Here's how the part is built. I have some questions about the finished solid (model axes, mm). Face numbers are marked on the shaded views. A direction names the side the tool comes from. Round coordinates to 2 decimals unless told otherwise and drop trailing zeros. Loops run counter-clockwise (first coordinate to the right, second up) from the corner with the lowest first, then second, coordinate; pieces in that order, holes last. Notation, with made-up numbers: (0.5, 5) -> (50.5, 5) arc R30 ccw to (50.5, 36) -> close; hole circle Ø8 at (45.5, 50.25). An arc over 180 degrees is marked (long way). One line per item, written item: value. Start each with the question number.
```python
from build123d import *

# Parameters (mm, degrees)
SKETCH2_R               = 4.3
SKETCH2_R_2             = 4
CUT_EXTRUDE_THIN1_DEPTH = 0.5
SKETCH3_R               = 3.5
SKETCH3_R_2             = 2.5
CUT_EXTRUDE1_DEPTH      = 0.2
SKETCH4_R               = 4
CUT_EXTRUDE2_DEPTH      = 0.1


with BuildPart() as part:
    # Sketch1 → Revolve1 (revolve)
    with BuildSketch(Plane.XY, mode=Mode.PRIVATE) as revolve1_sk:
        Polygon((-6.5, 3), (-6.5, 2), (-4.75, 0), (-6.5, -2), (-6.5, -3), (-2, -3), (-2, 3), align=None)
    revolve(revolve1_sk.sketch.rotate(Axis((0, 0, 0), (0, 1, 0)), 270), axis=Axis((0, 0, 0), (0, 1, 0)))

    # Sketch2 → Cut-Extrude-Thin1 (cut)
    with BuildSketch(Plane.XZ.offset(3)):
        Circle(SKETCH2_R)
        Circle(SKETCH2_R_2, mode=Mode.SUBTRACT)
    cut_extrude_thin1 = extrude(amount=-CUT_EXTRUDE_THIN1_DEPTH, mode=Mode.SUBTRACT)

    # Sketch3 → Cut-Extrude1 (cut)
    with BuildSketch(Plane.XZ.offset(3)):
        with Locations(Location((0, 0, 0), (0, 0, 270))):
            Circle(SKETCH3_R)
        with Locations(Location((0, 0, 0), (0, 0, 270))):
            Circle(SKETCH3_R_2, mode=Mode.SUBTRACT)
    cut_extrude1 = extrude(amount=-CUT_EXTRUDE1_DEPTH, mode=Mode.SUBTRACT)

    # Mirror1: Cut-Extrude-Thin1, Cut-Extrude1 across plane
    add(cut_extrude_thin1.mirror(Plane.ZX), mode=Mode.SUBTRACT)
    add(cut_extrude1.mirror(Plane.ZX), mode=Mode.SUBTRACT)

    # Sketch4 → Cut-Extrude2 (cut, symmetric)
    with BuildSketch(Plane(origin=(0, 0, 0), x_dir=(1, 0, 0), z_dir=(0, 1, 0))):
        with Locations(Location((0, 0, 0), (0, 0, 90))):
            Circle(SKETCH4_R)
    extrude(amount=CUT_EXTRUDE2_DEPTH, both=True, mode=Mode.SUBTRACT)


solid = part.part
```
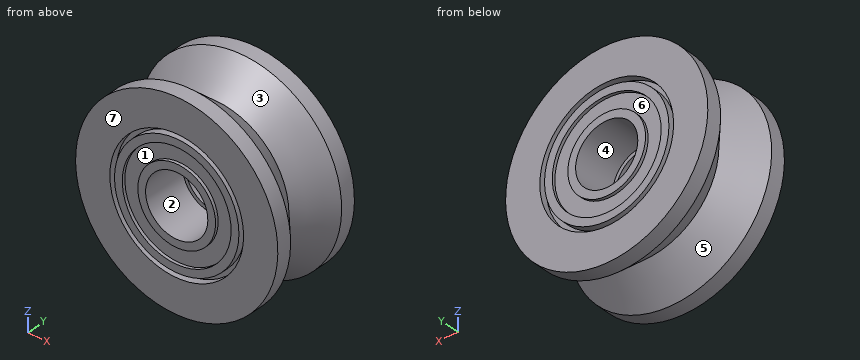
Q1. If we mould it in two halves opening along Z, with no side actions, what happens to the marked faces 4, 5, 6 and 7? For each: released by +Z, released by -Z, zero draft, split by the parting line, or undercut.
Q2. If I drill on line 1 along Y through (x, z) = (2.5, -0.5); line 2 along Y through (x, z) = (1.5, 1.5); line 3 along X through (y, z) = (2.7, 1.25), over which ranges is the centre line in solid material (lowest first)?
Q3. Which directions (+Z, -Z, +X, -X, +Y, -Y) give clear straight access to the entire face, cutting with the end or side of a thin tool? Please do the marked faces 1, 2 and 3.
Q4. I want a section at A-A on y = -2.2. Please give me the cut outline in (x, z).
Q5. Will these pins go through, and if not, where does the flat tip stop? P1, Ø1, axis at y = 0, z = 0, coming from the -X side; P2, Ø1.5, axis at y = -0.5, z = -2, coming from the -X side; P3, Ø3, axis at x = -3, y = 0, coming from the -Z side.
Answers below:
1. face 4: undercut
1. face 5: split by the parting line
1. face 6: undercut
1. face 7: zero draft
2. line 1: y = -2.8 to -0.1, 0.1 to 2.8
2. line 2: y = -3 to -0.1, 0.1 to 3
2. line 3: x = -6.38 to -4.11, -3.8 to -1.56, 1.56 to 3.8, 4.11 to 6.38
3. face 1: -Y
3. face 2: +Y, -Y
3. face 3: none
4. outline: circle Ø13 at (0, 0); hole circle Ø4 at (0, 0)
5. P1: stops at x = -5.19
5. P2: stops at x = -5.54
5. P3: stops at z = -5.45
